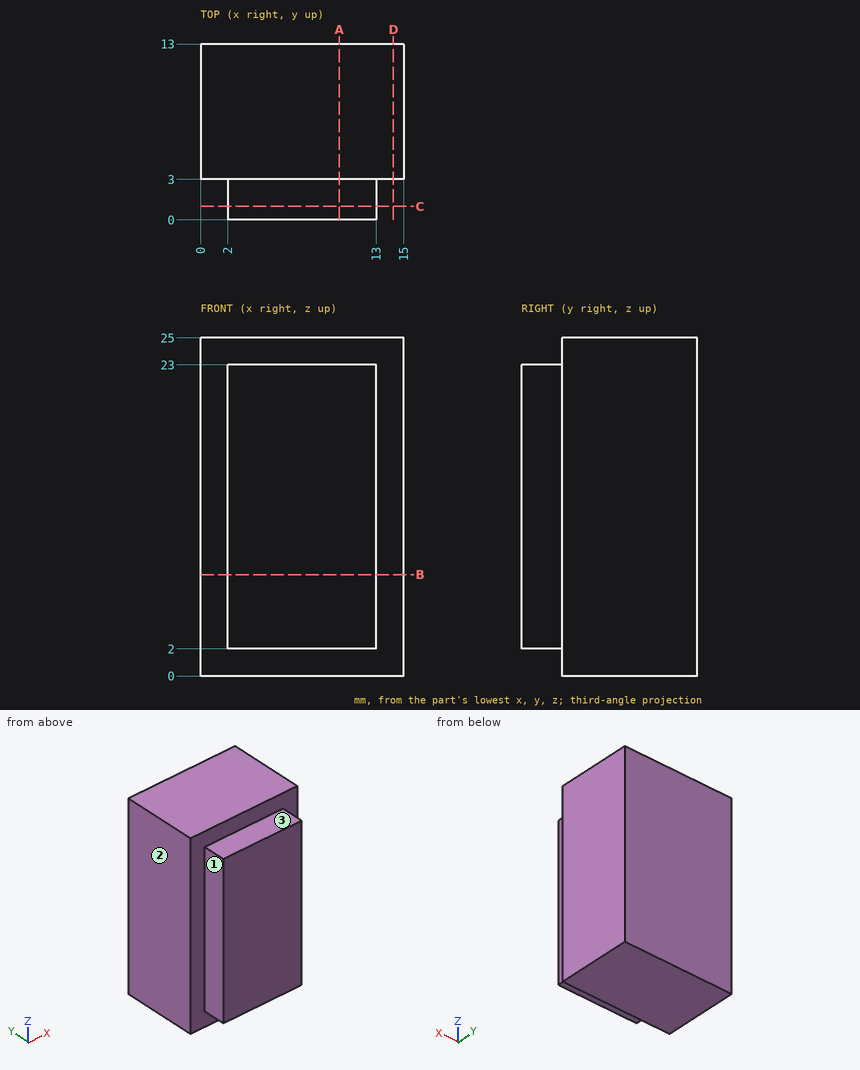
Answer from the drawing. Dimensions are ordinates in mm from the lowest x, y and z of the part. A direction names the side the tool comes from. Give positions to 0.01 mm unless a question says otherwise; leave off trailing zeros. Order: outer loops, then holes, each group sorted by start corner. A loop starts at its lowest first (then second) coordinate and runs counter-clockwise, first axis right, second up.
(1) Find section D-D (x = 14.25). Give the vertices of the cut face in (y, z), plus the area to 3 significant figures.
(2) For the marked faces 1, 2 and 3, determine the directions among +Z, -Z, +X, -X, +Y, -Y from which every point of the face is accessible in a straight line to the end or side of a thin tool.
(3) Find section C-C (y = 1). Give the vertices of the cut face in (x, z), plus the area to 3 significant figures.
(4) Find section A-A (x = 10.25). Give the vertices of the cut face in (y, z).
(5) Find section B-B (z = 7.5). Give the vertices of the cut face in (x, y), plus the area to 3 significant figures.
(6) Straight lines are drawn through the part: L1, parallel to X at y = 0.5, z = 13; L2, parallel to Y at x = 1.75, z = 1.5; L3, parallel to Z at x = 6.75, y = 1.25. For each, find the intervals that lie inside material, in ascending order.
(7) Given pin 1 (0.9 mm diameter, centred on y = 1.5, z = 12.5, fed in from +X); pin 2 (1.5 mm diameter, centred on x = 7.5, y = 1, fed in from -Z), each flat-ended and moving along its own axis, determine where each tip first touches the part or whether it passes through.
Result sheet:
1. outline: (3, 0) - (13, 0) - (13, 25) - (3, 25) - close
1. area: 250 mm2
2. face 1: +Z, -Z, -X, -Y
2. face 2: +Z, -Z, -X, +Y, -Y
2. face 3: +Z, +X, -X, -Y
3. outline: (2, 2) - (13, 2) - (13, 23) - (2, 23) - close
3. area: 231 mm2
4. outline: (0, 2) - (3, 2) - (3, 0) - (13, 0) - (13, 25) - (3, 25) - (3, 23) - (0, 23) - close
5. outline: (0, 3) - (2, 3) - (2, 0) - (13, 0) - (13, 3) - (15, 3) - (15, 13) - (0, 13) - close
5. area: 183 mm2
6. L1: x = 2 to 13
6. L2: y = 3 to 13
6. L3: z = 2 to 23
7. pin 1: stops at x = 13
7. pin 2: stops at z = 2
